Could you check a few things on this model? Use its own coordinates, in mm. Face numbers are marked on the shaded views. A direction names the side the tool comes from. Round coordinates to 2 decimals unless told otherwise and drop trailing zeros. Loops run counter-clockwise (first coordinate to the right, second up) from the corner with the lowest first, then second, coordinate; pieces in that order, holes last. Notation, with made-up numbers: (73, 68.5) -> (95, 68.5) arc R15 cw to (95, 81.5) -> close; hole circle Ø3 at (-20.75, -32.75). An arc over 180 degrees is marked (long way). One line per item, written item: value.
from build123d import *

# Parameters (mm, degrees)
SKETCH_2_R          = 2.65
SKETCH_2_R_2        = 12.1
EXTRUDE_1_DEPTH     = 7
SKETCH_3_R          = 12.1
SKETCH_3_R_2        = 11.6
EXTRUDE_2_DEPTH     = 1.9
FILLET_1_R          = 5
CUT_EXTRUDE_2_DEPTH = 1
CUT_EXTRUDE_3_DEPTH = 7
FILLET_3_R          = 1


with BuildPart() as part:
    # 草图2 → 凸台-拉伸1 (new body)
    with BuildSketch(Plane(origin=(0, 0, 0), x_dir=(1, 0, 0), z_dir=(0, 1, 0))):
        with BuildLine():
            Line((33.483093904, -23), (49.97, -23))
            ThreePointArc((49.97, -23), (54.919747468, -20.949747468), (56.97, -16))
            Line((56.97, -16), (56.97, 0))
            ThreePointArc((56.97, 0), (54.919747468, 4.949747468), (49.97, 7))
            Line((49.97, 7), (33.483093904, 7))
            ThreePointArc((33.483093904, 7), (24.985, 9.24), (16.486906096, 7))
            Line((16.486906096, 7), (0, 7))
            ThreePointArc((0, 7), (-4.949747468, 4.949747468), (-7, 0))
            Line((-7, 0), (-7, -16))
            ThreePointArc((-7, -16), (-4.949747468, -20.949747468), (0, -23))
            Line((0, -23), (16.486906096, -23))
            ThreePointArc((16.486906096, -23), (24.985, -25.24), (33.483093904, -23))
        make_face()
        Circle(SKETCH_2_R, mode=Mode.SUBTRACT)
        with Locations((0, -16)):
            Circle(SKETCH_2_R, mode=Mode.SUBTRACT)
        with Locations((49.97, 0)):
            Circle(SKETCH_2_R, mode=Mode.SUBTRACT)
        with Locations((49.97, -16)):
            Circle(SKETCH_2_R, mode=Mode.SUBTRACT)
        with Locations((24.985, -8)):
            Circle(SKETCH_2_R_2, mode=Mode.SUBTRACT)
    extrude(amount=EXTRUDE_1_DEPTH)

    # 草图3 → 凸台-拉伸2 (add)
    with BuildSketch(Plane(origin=(0, 7, 0), x_dir=(1, 0, 0), z_dir=(0, 1, 0))):
        with Locations((24.985, -8)):
            Circle(SKETCH_3_R)
        with Locations((24.985, -8)):
            Circle(SKETCH_3_R_2, mode=Mode.SUBTRACT)
    extrude(amount=-EXTRUDE_2_DEPTH)

    # 圆角1
    fillet_1_edges = [part.edges().sort_by_distance(p)[0] for p in [
        (16.486906096, 3.5, 23),
        (16.486906096, 3.5, -7),
        (33.483093904, 3.5, -7),
        (33.483093904, 3.5, 23),
    ]]
    fillet(fillet_1_edges, radius=FILLET_1_R)

    # 草图5 → 切除-拉伸2 (cut)
    with BuildSketch(Plane(origin=(0, 7, 0), x_dir=(1, 0, 0), z_dir=(0, 1, 0))):
        with BuildLine():
            Line((21.235, 8.827213079), (21.235, 2.977135328))
            ThreePointArc((21.235, 2.977135328), (24.985, 3.6), (28.735, 2.977135328))
            Line((28.735, 2.977135328), (28.735, 8.827213079))
            ThreePointArc((28.735, 8.827213079), (24.985, 9.24), (21.235, 8.827213079))
        make_face()
    extrude(amount=-CUT_EXTRUDE_2_DEPTH, mode=Mode.SUBTRACT)

    # 草图6 → 切除-拉伸3 (cut, through all)
    with BuildSketch(Plane(origin=(0, 6, 0), x_dir=(1, 0, 0), z_dir=(0, 1, 0))):
        with BuildLine():
            Line((28.735, 2.977135328), (28.735, 3.504238349))
            ThreePointArc((28.735, 3.504238349), (24.985, 4.1), (21.235, 3.504238349))
            Line((21.235, 3.504238349), (21.235, 2.977135328))
            ThreePointArc((21.235, 2.977135328), (24.985, 3.6), (28.735, 2.977135328))
        make_face()
    extrude(amount=-CUT_EXTRUDE_3_DEPTH, mode=Mode.SUBTRACT)

    # 圆角3
    fillet_3_edges = [part.edges().sort_by_distance(p)[0] for p in [
        (21.235, 6.5, -8.827213079),
        (28.735, 6.5, -8.827213079),
    ]]
    fillet(fillet_3_edges, radius=FILLET_3_R)


solid = part.part
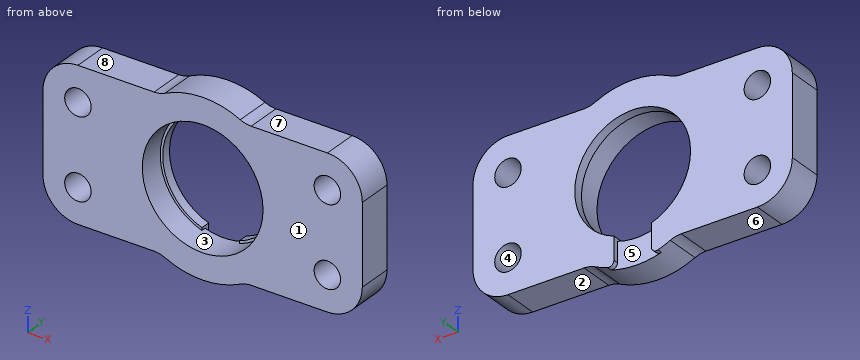
(1) If I drill on L1, parallel to Z at x = 0, y = 3; L2, parallel to X at y = 3.75, z = 16; L3, parallel to Z at x = 48, y = 6.5, over which ranges is the centre line in solid material (lowest first)?
Recorded:
L1: -7 to -2.65, 2.65 to 13.35, 18.65 to 23
L2: -7 to -2.65, 2.65 to 15.91, 34.06 to 47.32, 52.62 to 56.97
L3: -7 to -1.77, 1.77 to 14.23, 17.77 to 23
(2) If we section it at B-B, the plane y = 0.75: Please give me the cut outline in (x, z) (3 decimals).
Recorded:
outline: (-7, 0) arc R7 ccw to (0, -7) -> (15.258, -7) arc R5 cw to (17.445, -7.504) arc R17.24 ccw to (32.525, -7.504) arc R5 cw to (34.712, -7) -> (49.97, -7) arc R7 ccw to (56.97, 0) -> (56.97, 16) arc R7 ccw to (49.97, 23) -> (34.712, 23) arc R5 cw to (32.525, 23.504) arc R17.24 ccw to (17.445, 23.504) arc R5 cw to (15.258, 23) -> (0, 23) arc R7 ccw to (-7, 16) -> close; hole circle Ø5.3 at (0, 0); hole circle Ø5.3 at (0, 16); hole circle Ø24.2 at (24.985, 8); hole circle Ø5.3 at (49.97, 0); hole circle Ø5.3 at (49.97, 16)
(3) If we section it at A-A, the plane z = 8: Please give me the cut outline in (x, y) (3 decimals).
Recorded:
outline: (-7, 0) -> (12.885, 0) -> (12.885, 5.1) -> (13.385, 5.1) -> (13.385, 7) -> (-7, 7) -> close; (36.585, 5.1) -> (37.085, 5.1) -> (37.085, 0) -> (56.97, 0) -> (56.97, 7) -> (36.585, 7) -> close
(4) If we section it at C-C, the plane x = 26: Please give me the cut outline in (y, z), then the cut area to 3 significant figures.
Recorded:
outline: (0, -9.21) -> (6, -9.21) -> (6, -4.06) -> (0, -4.06) -> close; (0, 20.06) -> (5.1, 20.06) -> (5.1, 19.56) -> (7, 19.56) -> (7, 25.21) -> (0, 25.21) -> close
area: 67.9 mm²
(5) For the marked faces 5, 6, 7 and 8, which set-ups out of +Z, -Z, +X, -X, +Y, -Y let a thin tool reach every point of the face, with its end or its side?
Recorded:
face 5: -Z, +Y
face 6: -Z, -X, +Y, -Y
face 7: +Z, +X, +Y, -Y
face 8: +Z, -X, +Y, -Y
(6) I'm going to push flat-ended pins straight in: pin 1 Ø2 at (x, y) = (43, 4.5) entering from +Z; pin 2 Ø1 at (y, z) = (6, -5) entering from +X; pin 3 Ø0.6 at (y, z) = (6.5, -4) entering from -X. Where does each tip first touch, or does it pass through?
Recorded:
pin 1: z = 23
pin 2: x = 55.33
pin 3: x = -5.94
(7) Thinking about a two-plate mould opening in Z: for the marked faces 1, 2, 3 and 4, which applies, released by +Z, released by -Z, zero draft, split by the parting line, or undercut?
Recorded:
face 1: zero draft
face 2: released by -Z
face 3: undercut
face 4: undercut
(8) If we section it at D-D, the plane z = 3.5: Please give me the cut outline in (x, y), then the cut area to 3 significant figures.
Recorded:
outline: (-7, 0) -> (13.75, 0) -> (13.75, 5.1) -> (14.29, 5.1) -> (14.29, 7) -> (-7, 7) -> close; (35.68, 5.1) -> (36.22, 5.1) -> (36.22, 0) -> (56.97, 0) -> (56.97, 7) -> (35.68, 7) -> close
area: 293 mm²
